Build history of the part. All positions in model axes, mm. Face numbers are marked on the shaded views. A direction names the side the tool comes from. Coordinates: 2 decimals unless noted, no trailing zeros. Write each loop counter-clockwise with the first axis right and the second up, starting at its lowest first coordinate (ties: lowest second). Pieces come first, ordered by that corner, then holes. Notation, with made-up numbers: (77, 39) -> (95, 39) arc R35 ccw to (95, 76) -> close; hole circle Ø9 at (56, 36.5). An arc over 180 degrees is marked (long way). Write each question's results on one line, items separated by ' | '. Start each with the question number.
Q1. Saw through at B-B on y = -110. Give the cut face in (x, z), and give its area (3 significant figures).
Q2. Drop flat-ended pins along their axis: pin 1 Ø9 at (x, y) = (7, -105) entering from -Z; pin 2 Ø3.5 at (x, y) = (0.5, -42.5) entering from +Z. Give the stop position or say it passes through.
Q3. Drill centre lines: line 1 (X direction, y = -142.5, z = -15.25); line 2 (Z direction, x = 0, y = -20); line 3 (Z direction, x = -10, y = -132). Where is each one in solid material? Low to high.
Q4. Tool access for the marked faces 4 and 5: list every direction of +Z, -Z, +X, -X, +Y, -Y with a clear straight run to the whole face (end or side of a thin tool).
Q5. Two-plate mould, pull along X, no slides. Class the marked faces 1, 2 and 3: released by +X, released by -X, zero draft, split by the parting line, or undercut.
Q6. Saw through at A-A on z = -16. Give the cut face in (x, y).
Q7. Saw through at C-C on x = -12.5. Give the cut face in (y, z), and give its area (3 significant figures).
Q8. Saw through at D-D on x = -6.5. Give the cut face in (y, z).
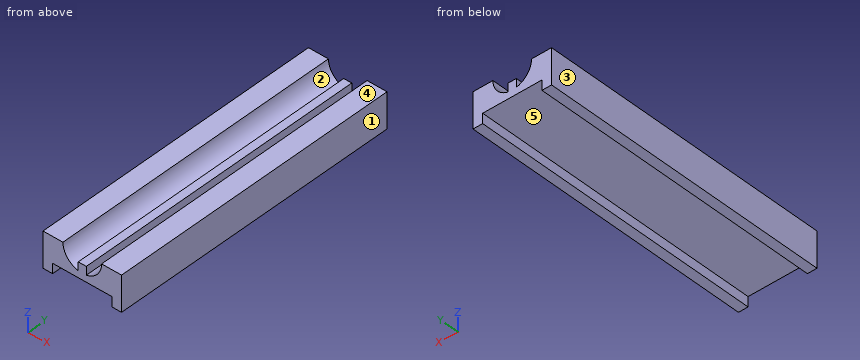
from build123d import *

# Parameters (mm, degrees)
F1_DEPTH = 150


with BuildPart() as f1:
    # F0 (on Front) → F1 (new body)
    with BuildSketch(Plane.XZ):
        with BuildLine():
            Line((15.1, -18), (20, -18))
            Line((20, -18), (20, 0))
            Line((20, 0), (9.84551, 0))
            ThreePointArc((9.84551, 0), (7.652364, -6.194787), (2.05, -9.629723))
            Line((2.05, -9.629723), (2.05, -5.346))
            Line((2.05, -5.346), (-2.05, -5.346))
            Line((-2.05, -5.346), (-2.05, -9.629723))
            ThreePointArc((-2.05, -9.629723), (-7.652364, -6.194787), (-9.84551, 0))
            Line((-9.84551, 0), (-20, 0))
            Line((-20, 0), (-20, -18))
            Line((-20, -18), (-15.1, -18))
            Line((-15.1, -18), (-15.1, -13))
            Line((-15.1, -13), (15.1, -13))
            Line((15.1, -13), (15.1, -18))
        make_face()
    extrude(amount=F1_DEPTH)


solid = f1.part
Returned:
1) outline: (-20, -18) -> (-15.1, -18) -> (-15.1, -13) -> (15.1, -13) -> (15.1, -18) -> (20, -18) -> (20, 0) -> (9.85, 0) arc R9.85 cw to (2.05, -9.63) -> (2.05, -5.35) -> (-2.05, -5.35) -> (-2.05, -9.63) arc R9.85 cw to (-9.85, 0) -> (-20, 0) -> close | area: 435 mm2
2) pin 1: stops at z = -13 | pin 2: stops at z = -5.35
3) line 1: x = -20 to -15.1, 15.1 to 20 | line 2: z = -13 to -5.35 | line 3: z = -13 to 0
4) face 4: +Z, +X, -X, +Y, -Y | face 5: -Z, +Y, -Y
5) face 1: released by +X | face 2: undercut | face 3: released by -X
6) outline: (-20, -150) -> (-15.1, -150) -> (-15.1, 0) -> (-20, 0) -> close; (15.1, -150) -> (20, -150) -> (20, 0) -> (15.1, 0) -> close
7) outline: (-150, -13) -> (0, -13) -> (0, 0) -> (-150, 0) -> close | area: 1,950 mm2
8) outline: (-150, -13) -> (0, -13) -> (0, -7.39) -> (-150, -7.39) -> close
